Design review of the part shown in the three views and the two pictorial views. Dimensions are in mm from the part's minimum x, y and z. A direction names the side the tool comes from. Coordinates: 2 decimals unless noted, no trailing zeros. Loops run counter-clockwise (first coordinate to the right, second up) from the corner with the lowest first, then second, coordinate; pieces in that order, holes last. Notation, with made-up numbers: (36.25, 17) -> (66.25, 17) arc R25 cw to (66.25, 50) -> close; hole circle Ø3 at (32.25, -10). An arc over 180 degrees is marked (long way). Answer in a Markdown table with one row per item.
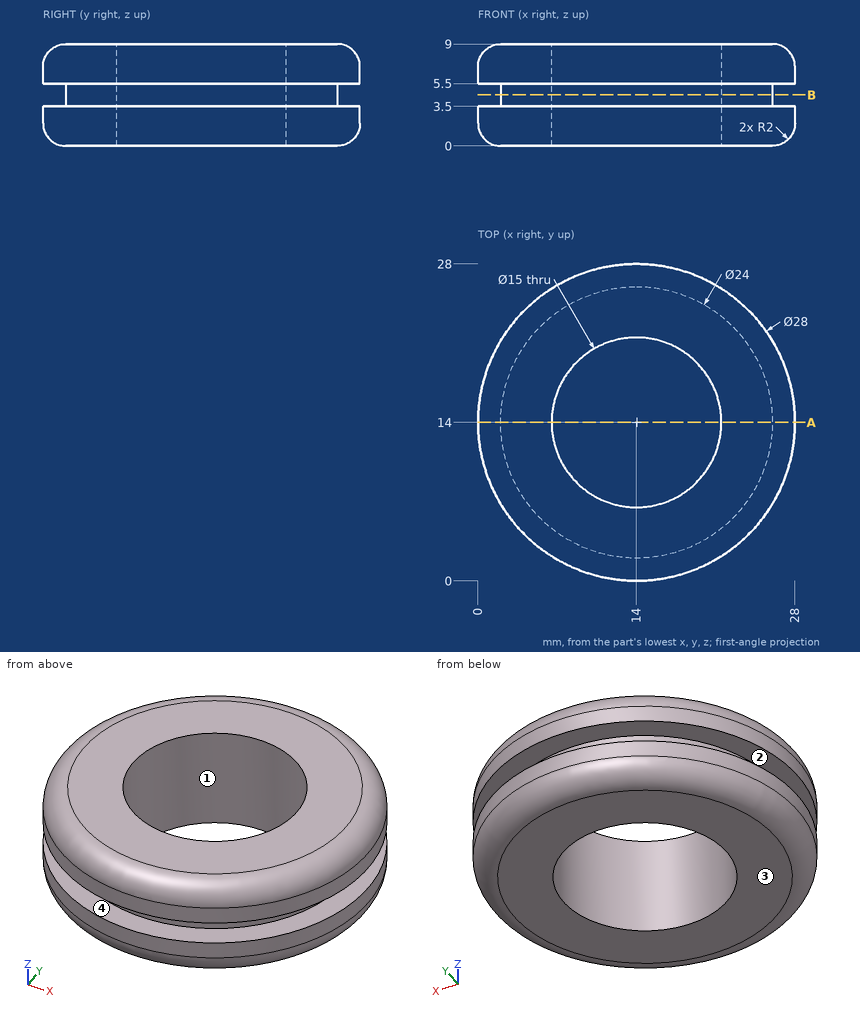
Item 1: Insertion check: pin 1 (14 mm diameter, centred on x = 14.5, y = 10, fed in from -Z); pin 2 (5 mm diameter, centred on x = 11, z = 2, fed in from -Y); pin 3 (1 mm diameter, centred on y = 3, z = 6.5, fed in from +X). Each pin has a flat end and moves straight along its axis. Give the tip position at first contact, or say it passes through.
Worked answers:
| item | result |
|---|---|
| pin 1 | z = 0 |
| pin 2 | y = 0.01 |
| pin 3 | x = 23.26 |
Item 2: For L1, parallel to Y at x = 14, z = 6; L2, parallel to Z at x = 24.25, y = 21.75; L3, parallel to Y at x = 15.5, z = 8.25, list the stretches that pass through material, from the lowest coordinate up.
Worked answers:
| item | result |
|---|---|
| L1 | 0 to 6.5, 21.5 to 28 |
| L2 | 0.19 to 3.5, 5.5 to 8.81 |
| L3 | 0.52 to 6.65, 21.35 to 27.48 |
Item 3: Take a section at B-B, the plane z = 4.5. State the section outline as (x, y) points, and give its area (3 significant figures).
Worked answers:
| item | result |
|---|---|
| outline | circle Ø24 at (14, 14); hole circle Ø15 at (14, 14) |
| area | 276 mm² |
Item 4: Take a section at A-A, the plane y = 14. State the section outline as (x, z) points, and give its area (3 significant figures).
Worked answers:
| item | result |
|---|---|
| outline | (0, 2) arc R2 ccw to (2, 0) -> (6.5, 0) -> (6.5, 9) -> (2, 9) arc R2 ccw to (0, 7) -> (0, 5.5) -> (2, 5.5) -> (2, 3.5) -> (0, 3.5) -> close; (21.5, 0) -> (26, 0) arc R2 ccw to (28, 2) -> (28, 3.5) -> (26, 3.5) -> (26, 5.5) -> (28, 5.5) -> (28, 7) arc R2 ccw to (26, 9) -> (21.5, 9) -> close |
| area | 106 mm² |
Item 5: For the marked faces 3 and 4, list the 3-axis set-ups (+Z, -Z, +X, -X, +Y, -Y) from which the entire face can be reached by the end or side of a thin tool; tool diameter is ignored.
Worked answers:
| item | result |
|---|---|
| face 3 | -Z, +X, -X, +Y, -Y |
| face 4 | none |
Item 6: The part is to be moulded in two halves that separate along Y. For the marked faces 1 and 2, say which applies: +Y half, -Y half, draft (parallel to the pull), parting line (faces both ways), or undercut.
Worked answers:
| item | result |
|---|---|
| face 1 | undercut |
| face 2 | draft |
